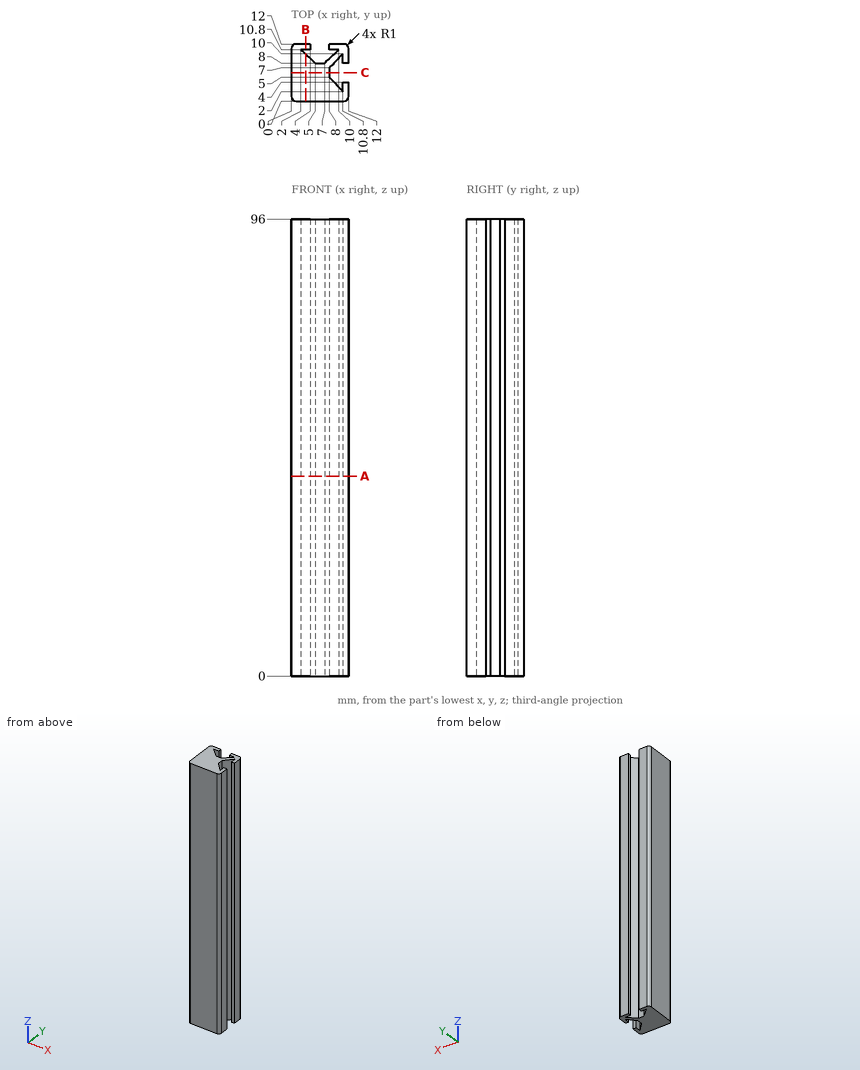
Geometry check sheet. Reference: drawing and pictorial views, mm from the part's lowest x, y, z. Give positions to 0.01 mm unless a question says otherwise; leave off trailing zeros. Order: outer loops, then holes, each group sorted by start corner. A loop starts at its lowest first (then second) coordinate and runs counter-clockwise, first axis right, second up. Notation, with made-up numbers: M 71,46 L 125,46 A24 ccw 125,79 Z; hole C 11.25,27.25 d1. An arc over 180 degrees is marked long. Answer in a Markdown table with one row per item. Add a question column.
Q1. Sectioned sample at B-B, the plane x = 3. Record the boundary of the cut face in (y, z), and give its area (3 significant figures).
Q2. Sectioned sample at C-C, the plane y = 6. Record the boundary of the cut face in (x, z), and give its area (3 significant figures).
Q3. Sectioned sample at A-A, the plane z = 42. Record the boundary of the cut face in (x, y), and give its area (3 significant figures).
Q4. Gauge pin test, flat ends, axial feed: pin 1 Ø1 at (x, z) = (6, 46.5) entering from +Y; pin 2 Ø1 at (y, z) = (6, 30) entering from +X. Record the tip position at first contact, or that the pin passes through.
Q5. Thickness scan on L1, parallel to Y at x = 8.5, z = 7; L2, parallel to X at y = 9, z = 10.5. Record the ranges inside material, lowest first.
Verdict:
| question | item | result |
|---|---|---|
| 1 | outline | M 0,0 L 9.87,0 L 9.87,96 L 0,96 Z; M 10.8,0 L 12,0 L 12,96 L 10.8,96 Z |
| 1 | area | 1,060 mm² |
| 2 | outline | M 0,0 L 8,0 L 8,96 L 0,96 Z |
| 2 | area | 768 mm² |
| 3 | outline | M 0,1 A1 ccw 1,0 L 11,0 A1 ccw 12,1 L 12,4 L 10.8,4 L 10.8,2 L 8,5 L 8,7 L 10.8,10 L 10.8,8 L 12,8 L 12,11 A1 ccw 11,12 L 8,12 L 8,10.8 L 10,10.8 L 7,8 L 5,8 L 2,10.8 L 4,10.8 L 4,12 L 1,12 A1 ccw 0,11 Z |
| 3 | area | 106 mm² |
| 4 | pin 1 | y = 8 |
| 4 | pin 2 | x = 8 |
| 5 | L1 | 0 to 4.46, 7.54 to 9.4, 10.8 to 12 |
| 5 | L2 | 0 to 3.93, 8.07 to 9.87, 10.8 to 12 |
